The drawing under review shows one solid part. Ordinate dimensions are in mm from its lowest x, y, z. Give positions to 0.01 mm unless a question says otherwise; leave off trailing zeros. Order: outer loops, then holes, each group sorted by start corner. A loop starts at its lowest first (then second) coordinate and runs counter-clockwise, first axis right, second up. Notation, with made-up numbers: (7, 29) - (18, 29) arc R12 ccw to (18, 44) - close; hole circle Ø7 at (-5, 65). An arc over 180 degrees is marked (long way). Use CSV: the item, a comma, the result in double quotes. Start each with the question number.
1. Take a section at B-B, the plane y = 20. State the section outline as (x, z) points.
2. To check wall thickness, follow line 1 (Y direction, x = 172.5, z = 1.1); line 2 (X direction, y = 140, z = 0.85); line 3 (X direction, y = 7.5, z = 0.8). State the ranges of each line that lie inside material, in increasing order. Write a range as [from, to].
3. Take a section at A-A, the plane x = 7.5. State the section outline as (y, z) points, then the cut area to 3 significant figures.
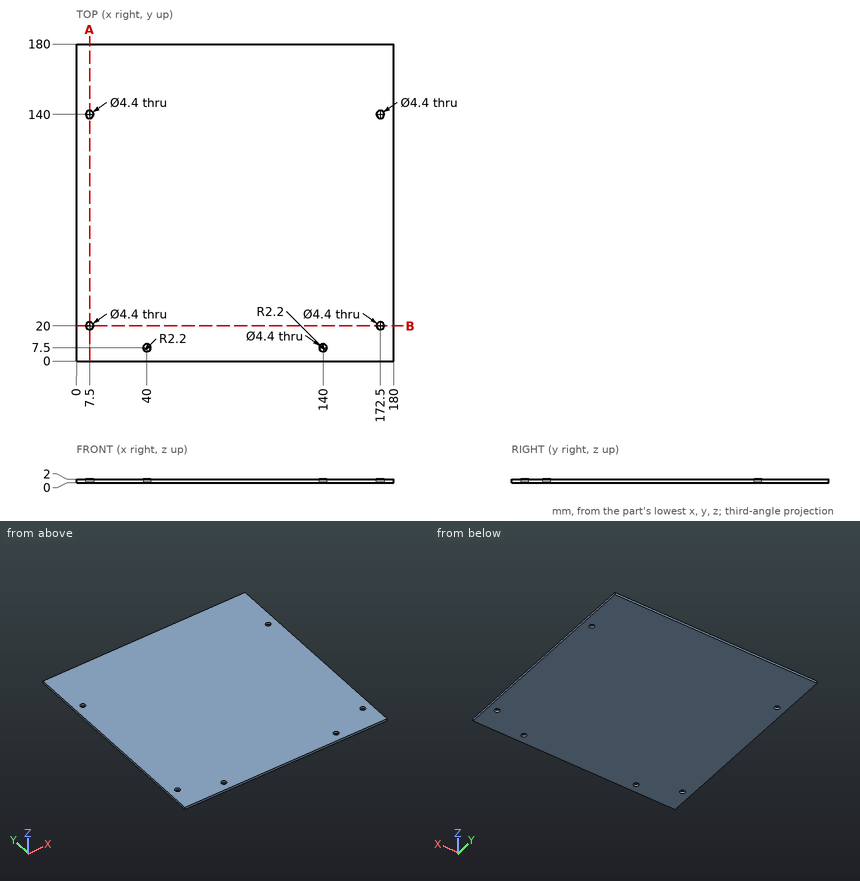
Determined:
1,outline,"(0, 0) - (5.3, 0) - (5.3, 2) - (0, 2) - close; (9.7, 0) - (170.3, 0) - (170.3, 2) - (9.7, 2) - close; (174.7, 0) - (180, 0) - (180, 2) - (174.7, 2) - close"
2,line 1,"y = [0, 17.8], [22.2, 137.8], [142.2, 180]"
2,line 2,"x = [0, 5.3], [9.7, 170.3], [174.7, 180]"
2,line 3,"x = [0, 37.8], [42.2, 137.8], [142.2, 180]"
3,outline,"(0, 0) - (17.8, 0) - (17.8, 2) - (0, 2) - close; (22.2, 0) - (137.8, 0) - (137.8, 2) - (22.2, 2) - close; (142.2, 0) - (180, 0) - (180, 2) - (142.2, 2) - close"
3,area,"342 mm²"
